Geometry: final body of the model. Coordinates: model frame, mm. Give positions to 0.01 mm unless a question says otherwise; leave off trailing zeros. Order: outer loops, then holes, each group sorted by start corner. A loop starts at its lowest first (then second) coordinate and runs counter-clockwise, first axis right, second up. Notation, with made-up numbers: M 83.25,-16 L 113.25,-16 A22 cw 113.25,-8 Z; hole C 36,68.5 d4. An arc over 180 degrees is marked long. Write item = value, one per line. Start each with the question number.
from build123d import *

# Parameters (mm, degrees)
F0_R     = 3
F0_R_2   = 2.5
F1_DEPTH = 300
F2_R     = 2
F3_R     = 7


# Not quite as in the source:
# - a feature names something its author has since deleted; it is built from what else it names


with BuildPart() as f1:
    # F0 (on Top) → F1 (new body)
    with BuildSketch(Plane.XY):
        with BuildLine():
            Line((18.15, -30), (30, -30))
            Line((30, -30), (30, -18.15))
            Line((30, -18.15), (27.5, -18.15))
            Line((27.5, -18.15), (27.5, -20.15))
            Line((27.5, -20.15), (21.5477069044, -20.15))
            ThreePointArc((21.5477069044, -20.15), (19.5, -15), (21.5477069044, -9.85))
            Line((21.5477069044, -9.85), (27.5, -9.85))
            Line((27.5, -9.85), (27.5, -11.85))
            Line((27.5, -11.85), (30, -11.85))
            Line((30, -11.85), (30, 11.85))
            Line((30, 11.85), (27.5, 11.85))
            Line((27.5, 11.85), (27.5, 9.85))
            Line((27.5, 9.85), (21.5477069044, 9.85))
            ThreePointArc((21.5477069044, 9.85), (19.5, 15), (21.5477069044, 20.15))
            Line((21.5477069044, 20.15), (27.5, 20.15))
            Line((27.5, 20.15), (27.5, 18.15))
            Line((27.5, 18.15), (30, 18.15))
            Line((30, 18.15), (30, 30))
            Line((30, 30), (18.15, 30))
            Line((18.15, 30), (18.15, 27.5))
            Line((18.15, 27.5), (20.15, 27.5))
            Line((20.15, 27.5), (20.15, 21.5477069044))
            ThreePointArc((20.15, 21.5477069044), (15, 19.5), (9.85, 21.5477069044))
            Line((9.85, 21.5477069044), (9.85, 27.5))
            Line((9.85, 27.5), (11.85, 27.5))
            Line((11.85, 27.5), (11.85, 30))
            Line((11.85, 30), (-11.85, 30))
            Line((-11.85, 30), (-11.85, 27.5))
            Line((-11.85, 27.5), (-9.85, 27.5))
            Line((-9.85, 27.5), (-9.85, 21.5477069044))
            ThreePointArc((-9.85, 21.5477069044), (-15, 19.5), (-20.15, 21.5477069044))
            Line((-20.15, 21.5477069044), (-20.15, 27.5))
            Line((-20.15, 27.5), (-18.15, 27.5))
            Line((-18.15, 27.5), (-18.15, 30))
            Line((-18.15, 30), (-30, 30))
            Line((-30, 30), (-30, 18.15))
            Line((-30, 18.15), (-27.5, 18.15))
            Line((-27.5, 18.15), (-27.5, 20.15))
            Line((-27.5, 20.15), (-21.5477069044, 20.15))
            ThreePointArc((-21.5477069044, 20.15), (-19.5, 15), (-21.5477069044, 9.85))
            Line((-21.5477069044, 9.85), (-27.5, 9.85))
            Line((-27.5, 9.85), (-27.5, 11.85))
            Line((-27.5, 11.85), (-30, 11.85))
            Line((-30, 11.85), (-30, -11.85))
            Line((-30, -11.85), (-27.5, -11.85))
            Line((-27.5, -11.85), (-27.5, -9.85))
            Line((-27.5, -9.85), (-21.5477069044, -9.85))
            ThreePointArc((-21.5477069044, -9.85), (-19.5, -15), (-21.5477069044, -20.15))
            Line((-21.5477069044, -20.15), (-27.5, -20.15))
            Line((-27.5, -20.15), (-27.5, -18.15))
            Line((-27.5, -18.15), (-30, -18.15))
            Line((-30, -18.15), (-30, -30))
            Line((-30, -30), (-18.15, -30))
            Line((-18.15, -30), (-18.15, -27.5))
            Line((-18.15, -27.5), (-20.15, -27.5))
            Line((-20.15, -27.5), (-20.15, -21.5477069044))
            ThreePointArc((-20.15, -21.5477069044), (-15, -19.5), (-9.85, -21.5477069044))
            Line((-9.85, -21.5477069044), (-9.85, -27.5))
            Line((-9.85, -27.5), (-11.85, -27.5))
            Line((-11.85, -27.5), (-11.85, -30))
            Line((-11.85, -30), (11.85, -30))
            Line((11.85, -30), (11.85, -27.5))
            Line((11.85, -27.5), (9.85, -27.5))
            Line((9.85, -27.5), (9.85, -21.5477069044))
            ThreePointArc((9.85, -21.5477069044), (15, -19.5), (20.15, -21.5477069044))
            Line((20.15, -21.5477069044), (20.15, -27.5))
            Line((20.15, -27.5), (18.15, -27.5))
            Line((18.15, -27.5), (18.15, -30))
        make_face()
        with Locations((-25, -25)):
            Circle(F0_R, mode=Mode.SUBTRACT)
        with Locations((-15, -15)):
            Circle(F0_R_2, mode=Mode.SUBTRACT)
        with Locations((25, -25)):
            Circle(F0_R, mode=Mode.SUBTRACT)
        with Locations((15, -15)):
            Circle(F0_R_2, mode=Mode.SUBTRACT)
        with Locations((-25, 25)):
            Circle(F0_R, mode=Mode.SUBTRACT)
        with Locations((-15, 15)):
            Circle(F0_R_2, mode=Mode.SUBTRACT)
        Polygon((-7, 22), (-7, 27.5), (0, 27.5), (7, 27.5), (7, 22), (10, 16), (10, 10), (16, 10), (22, 7), (27.5, 7), (27.5, 0), (27.5, -7), (22, -7), (16, -10), (10, -10), (10, -16), (7, -22), (7, -27.5), (0, -27.5), (-7, -27.5), (-7, -22), (-10, -16), (-10, -10), (-16, -10), (-22, -7), (-27.5, -7), (-27.5, 0), (-27.5, 7), (-22, 7), (-16, 10), (-10, 10), (-10, 16), align=None, mode=Mode.SUBTRACT)
        with Locations((15, 15)):
            Circle(F0_R_2, mode=Mode.SUBTRACT)
        with Locations((25, 25)):
            Circle(F0_R, mode=Mode.SUBTRACT)
    extrude(amount=F1_DEPTH)

    # F2
    f2_edges = [f1.edges().sort_by_distance(p)[0] for p in [
        (-7, 27.5, 150),
        (7, 27.5, 150),
    ]]
    fillet(f2_edges, radius=F2_R)

    # F3
    f3_edges = [f1.edges().sort_by_distance(p)[0] for p in [
        (-10, 16, 150),
        (10, 16, 150),
    ]]
    fillet(f3_edges, radius=F3_R)


solid = f1.part
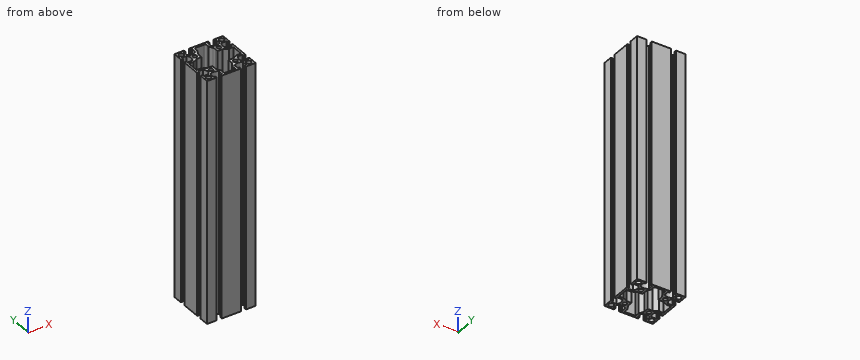
1) Cut plane A-A (y = -25). Return loops of the section in (x, z).
2) Ray query, L1, parallel to Y at x = 25, z = 102; L2, parallel to Y at x = -15, z = 211; L3, parallel to X at y = -24.5, z = 179. Return the intervals inside material, ascending.
3) Cut plane D-D (z = 277.5). Give the number of separate pieces and of enclosed holes in the cut face, plus the area to 3 significant figures.
4) Cut plane B-B (x = 0). Return loops of the section in (y, z).
5) Pin query (flat end, axial travel): pin 1 Ø6.5 at (y, z) = (-14, 128.5) entering from +X; pin 2 Ø2 at (y, z) = (-17, 134) entering from +X. Return the tip coordinate at first contact, or that it passes through.
Reply:
q1.outline = M -30,0 L -28,0 L -28,300 L -30,300 Z; M -22,0 L -20.15,0 L -20.15,300 L -22,300 Z; M -9.85,0 L -7,0 L -7,300 L -9.85,300 Z; M 7,0 L 9.85,0 L 9.85,300 L 7,300 Z; M 20.15,0 L 22,0 L 22,300 L 20.15,300 Z; M 28,0 L 30,0 L 30,300 L 28,300 Z
q2.L1 = -30 to -28, -22 to -20.15, -9.85 to -7, 7 to 9.85, 20.15 to 22, 28 to 30
q2.L2 = -19.5 to -17.5, -12.5 to -10, 10 to 12.5, 17.5 to 19.5
q2.L3 = -30 to -27.96, -22.04 to -20.15, -9.85 to -7, 7 to 9.85, 20.15 to 22.04, 27.96 to 30
q3.separate_pieces = 1
q3.enclosed_holes = 9
q3.area = 1,080 mm²
q4.outline = M -30,0 L -27.5,0 L -27.5,300 L -30,300 Z; M 27.5,0 L 30,0 L 30,300 L 27.5,300 Z
q5.pin_1 = 30
q5.pin_2 = 20.13
